Verification items for the finished model (mm, model axes). A direction names the side the tool comes from. Coordinates: 2 decimals unless noted, no trailing zeros. Loops run counter-clockwise (first coordinate to the right, second up) from the corner with the lowest first, then second, coordinate; pieces in that order, holes last. Notation, with made-up numbers: (86, -5) -> (143, -5) arc R13 ccw to (143, 7) -> close; hole circle Ø4 at (-35.5, 15.5). An arc over 180 degrees is marked (long way). Use CSV: the item, a comma, the result in double quotes. Start each with the question number.
```python
from build123d import *

# Parameters (mm, degrees)
F0_W     = 55
F0_H     = 25
F1_DEPTH = 13
F3_DEPTH = 16
F4_W     = 4.1
F4_H     = 4.2
F5_DEPTH = 31.6
F6_W     = 55
F6_H     = 10
F7_DEPTH = 5
F8_DEPTH = 3.5
F9_DEPTH = 3.5


with BuildPart() as f1:
    # F0 (on Top) → F1 (new body)
    with BuildSketch(Plane.XY):
        with Locations((19.0712029868, -0.8496874943)):
            Rectangle(F0_W, F0_H)
    extrude(amount=F1_DEPTH)

    # F2 (on face) → F3 (cut)
    with BuildSketch(Plane.XZ.offset(13.3496874943)):
        with BuildLine():
            Line((-1.9287970132, 6.5), (-1.9287970132, 9.1))
            ThreePointArc((-1.9287970132, 9.1), (-3.7672746443, 8.3384776311), (-4.5287970132, 6.5))
            Line((-4.5287970132, 6.5), (-1.9287970132, 6.5))
        make_face()
        with BuildLine():
            ThreePointArc((0.6712029868, 6.5), (-0.0903193822, 8.3384776311), (-1.9287970132, 9.1))
            Line((-1.9287970132, 9.1), (-1.9287970132, 6.5))
            Line((-1.9287970132, 6.5), (-4.5287970132, 6.5))
            ThreePointArc((-4.5287970132, 6.5), (-1.9287970132, 3.9), (0.6712029868, 6.5))
        make_face()
        with BuildLine():
            ThreePointArc((42.6712029868, 6.5), (41.9096806178, 8.3384776311), (40.0712029868, 9.1))
            Line((40.0712029868, 9.1), (40.0712029868, 6.5))
            Line((40.0712029868, 6.5), (42.6712029868, 6.5))
        make_face()
        with BuildLine():
            Line((40.0712029868, 6.5), (40.0712029868, 9.1))
            ThreePointArc((40.0712029868, 9.1), (38.2327253557, 4.6615223689), (42.6712029868, 6.5))
            Line((42.6712029868, 6.5), (40.0712029868, 6.5))
        make_face()
    extrude(amount=-F3_DEPTH, mode=Mode.SUBTRACT)

    # F4 (on face) → F5 (cut)
    with BuildSketch(Plane.XY.offset(13)):
        Polygon((35.9712029868, -6.6496874943), (35.9712029868, -10.8496874943), (40.0712029868, -10.8496874943), (44.1712029868, -10.8496874943), (44.1712029868, -6.6496874943), (40.0712029868, -6.6496874943), align=None)
        with Locations((0.1212029868, -8.7496874943)):
            Rectangle(F4_W, F4_H)
        with Locations((-3.9787970132, -8.7496874943)):
            Rectangle(F4_W, F4_H)
    extrude(amount=-F5_DEPTH, mode=Mode.SUBTRACT)

    # F6 (on face) → F7 (join)
    with BuildSketch(Plane.XY.offset(13)):
        with BuildLine():
            Line((-8.4287970132, 21.6503125057), (-8.4287970132, 11.6503125057))
            Line((-8.4287970132, 11.6503125057), (46.5712029868, 11.6503125057))
            Line((46.5712029868, 11.6503125057), (46.5712029868, 21.6503125057))
            Line((46.5712029868, 21.6503125057), (39.1712029868, 21.6503125057))
            ThreePointArc((39.1712029868, 21.6503125057), (36.5712029868, 19.0503125057), (33.9712029868, 21.6503125057))
            Line((33.9712029868, 21.6503125057), (4.1712029868, 21.6503125057))
            ThreePointArc((4.1712029868, 21.6503125057), (1.5712029868, 19.0503125057), (-1.0287970132, 21.6503125057))
            Line((-1.0287970132, 21.6503125057), (-8.4287970132, 21.6503125057))
        make_face()
        with Locations((19.0712029868, 6.6503125057)):
            Rectangle(F6_W, F6_H)
        with BuildLine():
            Line((-8.4287970132, 31.6503125057), (-8.4287970132, 21.6503125057))
            Line((-8.4287970132, 21.6503125057), (-1.0287970132, 21.6503125057))
            ThreePointArc((-1.0287970132, 21.6503125057), (1.5712029868, 24.2503125057), (4.1712029868, 21.6503125057))
            Line((4.1712029868, 21.6503125057), (33.9712029868, 21.6503125057))
            ThreePointArc((33.9712029868, 21.6503125057), (36.5712029868, 24.2503125057), (39.1712029868, 21.6503125057))
            Line((39.1712029868, 21.6503125057), (46.5712029868, 21.6503125057))
            Line((46.5712029868, 21.6503125057), (46.5712029868, 31.6503125057))
            Line((46.5712029868, 31.6503125057), (-8.4287970132, 31.6503125057))
        make_face()
    extrude(amount=F7_DEPTH)

    # F8 (add): a face of the model
    f8_faces = [f1.faces().sort_by_distance(p)[0] for p in [
        (19.0712029868, 16.5182016052, 18),
    ]]
    extrude(f8_faces, amount=F8_DEPTH)

    # F9 (cut): a face of the model
    f9_faces = [f1.faces().sort_by_distance(p)[0] for p in [
        (19.0712029868, 21.6503125057, 13),
    ]]
    extrude(f9_faces, amount=-F9_DEPTH, mode=Mode.SUBTRACT)


solid = f1.part
```
1. Cross-section at A-A, the plane y = -4.5. Record the boundary of the cut face in (x, z).
2. Cross-section at C-C, the plane z = 2. Record the boundary of the cut face in (x, y).
3. Scan lines: line 1 (X direction, y = -12.45, z = 6.5); line 2 (Y direction, x = 38, z = 11.25); line 3 (X direction, y = -8.5, z = 4). Record each from-to range of solid material in increasing order.
4. Depth check by flat-ended pin: pin 1 (5 mm diameter, centred on x = 12, z = 10, fed in from +Y); pin 2 (7 mm diameter, centred on x = 1.57, y = 21.65, fed in from -Z); pin 3 (3 mm diameter, centred on x = 36.57, y = 21.65, fed in from -Z); pin 4 (4 mm diameter, centred on x = 31, z = 15.5, fed in from -Y). Enter the tip coordinate at first touch or a pass-through.
5. Cross-section at B-B, the plane x = -3. Record the boundary of the cut face in (y, z).
6. Set-up check for faces 1 (the flat face through (19, -1, 0)), 2 (the flat face through (40, 2.65, 7)), 3 (the flat face through (43, -10.85, 7)), 4 (the flat face through (19, 11.65, 8)), 5 (the flat face through (19, -6, 13)): record each of +Z, -Z, +X, -X, +Y, -Y from which the full face is reachable in a straight line by a thin tool's end or side.
7. Release check for a two-part mould opening along X. For faces 6 (the flat face through (19, 22, 16.5)), 7 (the flat face through (-8.429, 4, 11)), 8 (the flat face through (-2, 2.65, 7)) record: released by +X, released by -X, zero draft, split by the parting line, or undercut.
8. Cross-section at D-D, the plane x = 8. Record the boundary of the cut face in (y, z), plus the area to 3 significant figures.
Solution:
1,outline,"(-8.43, 0) -> (46.57, 0) -> (46.57, 13) -> (-8.43, 13) -> close; hole circle Ø5.2 at (-1.93, 6.5); hole circle Ø5.2 at (40.07, 6.5)"
2,outline,"(-8.43, -13.35) -> (46.57, -13.35) -> (46.57, 11.65) -> (-8.43, 11.65) -> close; hole (-6.03, -10.85) -> (2.17, -10.85) -> (2.17, -6.65) -> (-6.03, -6.65) -> close; hole (35.97, -10.85) -> (44.17, -10.85) -> (44.17, -6.65) -> (35.97, -6.65) -> close"
3,line 1,"x = -8.43 to -4.53, 0.67 to 37.47, 42.67 to 46.57"
3,line 2,"y = -13.35 to -10.85, -6.65 to 11.65"
3,line 3,"x = -8.43 to -6.03, 2.17 to 35.97, 44.17 to 46.57"
4,pin 1,"stops at y = 11.65"
4,pin 2,"stops at z = 16.5"
4,pin 3,"passes through"
4,pin 4,"stops at y = 1.65"
5,outline,"(-13.35, 0) -> (-10.85, 0) -> (-10.85, 4.13) -> (-13.35, 4.13) -> close; (-13.35, 8.87) -> (-10.85, 8.87) -> (-10.85, 13) -> (-13.35, 13) -> close; (-6.65, 0) -> (11.65, 0) -> (11.65, 16.5) -> (31.65, 16.5) -> (31.65, 21.5) -> (1.65, 21.5) -> (1.65, 13) -> (-6.65, 13) -> (-6.65, 8.87) -> (2.65, 8.87) -> (2.65, 4.13) -> (-6.65, 4.13) -> close"
6,face 1,"-Z, +X, -X, +Y, -Y"
6,face 2,"-Y"
6,face 3,"+Z, -Z"
6,face 4,"-Z, +X, -X, +Y"
6,face 5,"+Z, +X, -X, -Y"
7,face 6,"zero draft"
7,face 7,"released by -X"
7,face 8,"undercut"
8,outline,"(-13.35, 0) -> (11.65, 0) -> (11.65, 16.5) -> (31.65, 16.5) -> (31.65, 21.5) -> (1.65, 21.5) -> (1.65, 13) -> (-13.35, 13) -> close"
8,area,"510 mm2"
